Autodesk Inventor part; units mm, degrees
ref_plane "YZ Plane" through (0, 0, 0) normal (1, 0, 0) x (0, 1, 0)
ref_plane "XZ Plane" through (0, 0, 0) normal (0, 1, 0) x (-1, 0, 0)
ref_plane "XY Plane" through (0, 0, 0) normal (0, 0, 1) x (1, 0, 0)
sketch "Boceto1" plane through (0, 0, 0) normal (0, 0, 1) x (1, 0, 0)
  line L0 (261.2, -146.2) -> (-261.2, -146.2)
  line L1 (-261.2, -146.2) -> (-261.2, 146.2)
  line L2 (-261.2, 146.2) -> (261.2, 146.2)
  line L3 (261.2, 146.2) -> (261.2, -146.2)
  line L4 (261.2, -146.2) -> (-261.2, 146.2) construction
  line L5 (-261.2, -146.2) -> (261.2, 146.2) construction
  line L6 (250, -135) -> (-250, -135)
  line L7 (-250, -135) -> (-250, 135)
  line L8 (-250, 135) -> (250, 135)
  line L9 (250, 135) -> (250, -135)
  line L10 (250, -135) -> (-250, 135) construction
  line L11 (-250, -135) -> (250, 135) construction
  point P0 (0, 0)
  dimension "d0" = 522.4
  dimension "d1" = 292.4
  dimension "d2" = 500
  dimension "d3" = 270
extrude "Extrusión1" add sketch "Boceto1" along normal blind 1.2
sketch "Boceto2" plane through (0, 0, 1.2) normal (0, 0, 1) x (1, 0, 0)
  line L0 (261.2, 146.2) -> (-261.2, 146.2)
  line L1 (-261.2, 146.2) -> (-261.2, -146.2)
  line L2 (261.2, -146.2) -> (261.2, 146.2)
  line L3 (-261.2, -146.2) -> (261.2, -146.2)
  line L4 (-260, 145) -> (260, 145)
  line L5 (260, 145) -> (260, -145)
  line L6 (260, -145) -> (-260, -145)
  line L7 (-260, -145) -> (-260, 145)
  point P0 (0, 0)
  dimension "d6" = 1.2
extrude "Extrusión2" add sketch "Boceto2" along normal blind 40
sketch "Boceto3" plane through (-261.2, -146.2, 0) normal (-1, 0, 0) x (0, 0, 1)
  line L0 (41.2, 292.4) -> (41.2, 0)
  line L1 (0, 292.4) -> (0, 0)
  line L2 (0, 0) -> (41.2, 0)
  line L3 (41.2, 292.4) -> (41.2, 0)
  line L4 (0, 292.4) -> (41.2, 292.4)
  circle A0 centre (20.6, 146.2) radius 10
  line L5 (10.6, 191.2) -> (30.6, 191.2)
  line L6 (30.6, 191.2) -> (30.6, 101.2)
  line L7 (30.6, 101.2) -> (10.6, 101.2)
  line L8 (10.6, 101.2) -> (10.6, 191.2)
  line L9 (10.6, 191.2) -> (30.6, 101.2) construction
  line L10 (30.6, 191.2) -> (10.6, 101.2) construction
  circle A1 centre (20.6, 191.2) radius 2.5
  circle A2 centre (20.6, 101.2) radius 2.5
  point P0 (0, 146.2)
  dimension "d9" = 20
  dimension "d12" = 90
  dimension "d13" = 5
  dimension "d14" = 5
extrude "Extrusión3" cut sketch "Boceto3" against normal blind 1000 contours A0
extrude "Extrusión4" cut sketch "Boceto3" against normal blind 1000 contours A1 L5 | L5 A1 | A2 L7 | L7 A2
properties part number "marco_ir"
Here's how the part is built. I have some questions about the finished solid (model axes, mm). A direction names the side the tool comes from. Give positions to 0.01 mm unless a question says otherwise; leave off trailing zeros. Write each loop counter-clockwise with the first axis right and the second up, starting at its lowest first coordinate (ties: lowest second). Pieces come first, ordered by that corner, then holes. Notation, with made-up numbers: (62, 71) -> (92, 71) arc R32 ccw to (92, 109) -> close; hole circle Ø11 at (24, 88.25). An arc over 180 degrees is marked (long way). Use one line per item in the form item = value.
1) Suppose I cut it at B-B (x = -12.5). Please give me the cut outline in (y, z), and give its area (3 significant figures).
Verdict:
outline = (-146.2, 0) -> (-135, 0) -> (-135, 1.2) -> (-145, 1.2) -> (-145, 41.2) -> (-146.2, 41.2) -> close; (135, 0) -> (146.2, 0) -> (146.2, 41.2) -> (145, 41.2) -> (145, 1.2) -> (135, 1.2) -> close
area = 123 mm2
2) Suppose I cut it at A-A (y = 97.5). Please give me the cut outline in (x, z).
Verdict:
outline = (-261.2, 0) -> (-250, 0) -> (-250, 1.2) -> (-260, 1.2) -> (-260, 41.2) -> (-261.2, 41.2) -> close; (250, 0) -> (261.2, 0) -> (261.2, 41.2) -> (260, 41.2) -> (260, 1.2) -> (250, 1.2) -> close
3) Suppose I cut it at C-C (y = 0). Please give me the cut outline in (x, z), and give its area (3 significant figures).
Verdict:
outline = (-261.2, 0) -> (-250, 0) -> (-250, 1.2) -> (-260, 1.2) -> (-260, 10.6) -> (-261.2, 10.6) -> close; (-261.2, 30.6) -> (-260, 30.6) -> (-260, 41.2) -> (-261.2, 41.2) -> close; (250, 0) -> (261.2, 0) -> (261.2, 10.6) -> (260, 10.6) -> (260, 1.2) -> (250, 1.2) -> close; (260, 30.6) -> (261.2, 30.6) -> (261.2, 41.2) -> (260, 41.2) -> close
area = 74.9 mm2
4) We'd pull the mould along Y, two halves only. Please class faces 1 (the face through (261.2, 2, 7)), 2 (the face through (-4, 146.2, 20)), 3 (the face through (-78, -139, 1.2)): +Y half, -Y half, draft (parallel to the pull), parting line (faces both ways), or undercut.
Verdict:
face_1 = draft
face_2 = +Y half
face_3 = undercut
5) If I drill on L1, parallel to Y at x = 260.35, z = 20.6; L2, parallel to X at y = -38.5, z = 16; L3, parallel to Y at x = -192, z = 7, over which ranges is the centre line in solid material (lowest first)? Write a range as [from, to].
Verdict:
L1 = [-146.2, -47.5], [-42.5, -10], [10, 42.5], [47.5, 146.2]
L2 = [-261.2, -260], [260, 261.2]
L3 = [-146.2, -145], [145, 146.2]
6) On a 3-axis mill with a long thin cutter (end or side, diameter ignored), from which of +Z, -Z, +X, -X, +Y, -Y can I reach the whole of each face in a straight line? I mean faces 4 (the face through (-260, -2, 8)), 5 (the face through (4, -146.2, 20)). Say none if no direction works.
Verdict:
face_4 = +Z
face_5 = +Z, -Z, +X, -X, -Y
